Geometry: final body of the model. Coordinates: model frame, mm. A direction names the side the tool comes from. Coordinates: 2 decimals unless noted, no trailing zeros. Loops run counter-clockwise (first coordinate to the right, second up) from the corner with the lowest first, then second, coordinate; pieces in that order, holes last. Notation, with made-up numbers: M 85,-27.5 L 120,-27.5 A30 cw 120,-0.5 Z; hole C -25.5,-27 d3. An arc over 180 degrees is marked long. Write each question's results on one line, items separated by ' | '. Start each with the question number.
from build123d import *

# Parameters (mm, degrees)
EXTRUDE_1_DEPTH = 8
SKETCH_2_R      = 5
EXTRUDE_2_DEPTH = 150
CHAMFER_1_SIZE  = 2
CHAMFER_1_SIZE2 = 1.154700538


with BuildPart() as part:
    # Эскиз1 → Бобышка-Вытянуть1 (new body)
    with BuildSketch(Plane(origin=(0, 0, 0), x_dir=(1, 0, 0), z_dir=(0, 1, 0))):
        Polygon((8.5, -4.907477288), (8.5, 4.907477288), (0, 9.814954576), (-8.5, 4.907477288), (-8.5, -4.907477288), (0, -9.814954576), align=None)
    extrude(amount=EXTRUDE_1_DEPTH)

    # Эскиз2 → Бобышка-Вытянуть2 (add)
    with BuildSketch(Plane(origin=(0, 8, 0), x_dir=(1, 0, 0), z_dir=(0, 1, 0))):
        Circle(SKETCH_2_R)
    extrude(amount=EXTRUDE_2_DEPTH)

    # Фаска1
    chamfer_1_edges = [part.edges().sort_by_distance(p)[0] for p in [
        (-4.25, 0, 7.361215932),
        (-8.5, 0, 0),
        (-4.25, 0, -7.361215932),
        (4.25, 0, -7.361215932),
        (8.5, 0, 0),
        (4.25, 0, 7.361215932),
    ]]
    chamfer_1_side = [part.faces().sort_by_distance(p)[0] for p in [
        (0, 0, 0),
    ]]
    chamfer(chamfer_1_edges, length=CHAMFER_1_SIZE, length2=CHAMFER_1_SIZE2, reference=chamfer_1_side[0])


solid = part.part
Item 1: Ray query, L1, parallel to Y at x = 6.25, z = 0; L2, parallel to X at y = 77.5, z = 0.5; L3, parallel to Z at x = -2, y = 41. Return the intervals inside material, ascending. Write a range as [from, to].
Item 2: Contact query for flat-ended pins moving along their axis: P1, Ø10, axis at y = 132, z = 6, coming from the +X side; P2, Ø6, axis at x = 5, y = 70, coming from the +Z side; P3, Ø3, axis at x = -1.5, y = 136, coming from the +Z side. Output: stop coordinate, or through.
Item 3: Set-up query: faces 1 (the flat face through (4, 8, 4)), 2 (the flat face through (0, 0, 0)). Return all of +Z, -Z, +X, -X, +Y, -Y with unobstructed straight access to the full face (end or side cutting, diameter ignored); none if empty.
Item 4: Section A-A, the plane z = 0. Return loops of the section in (x, y).
Item 5: Section B-B, the plane y = 66.5. Return loops of the section in (x, z), plus the area to 3 significant figures.
Solutions:
1) L1: y = [0, 8] | L2: x = [-4.97, 4.97] | L3: z = [-4.58, 4.58]
2) P1: stops at x = 4.9 | P2: stops at z = 4.58 | P3: stops at z = 5
3) face 1: +Y | face 2: +Z, -Z, +X, -X, -Y
4) outline: M -8.5,1.15 L -6.5,0 L 6.5,0 L 8.5,1.15 L 8.5,8 L 5,8 L 5,158 L -5,158 L -5,8 L -8.5,8 Z
5) outline: C 0,0 d10 | area: 78.5 mm²
